```python
from build123d import *

# Parameters (mm, degrees)
F0_W     = 650
F0_H     = 950
F1_DEPTH = 50
F4_DEPTH = 50


with BuildPart() as f1:
    # F0 (on Top) → F1 (new body)
    with BuildSketch(Plane.XY):
        Rectangle(F0_W, F0_H)
    extrude(amount=F1_DEPTH)

    # F3 (on offset) → F4 (join)
    with BuildSketch(Plane.XZ.offset(375)):
        Polygon((0, -158.604646672), (-86.0232526704, -97.1594661932), (-300, -250), (-127.9534946591, -250), align=None)
        Polygon((0, -35.7142857143), (-86.0232526704, -97.1594661932), (0, -158.604646672), (86.0232526704, -97.1594661932), align=None)
        Polygon((50, 0), (0, -35.7142857143), (86.0232526704, -97.1594661932), (222.0465053409, 0), align=None)
        Polygon((-50, 0), (-222.0465053409, 0), (-86.0232526704, -97.1594661932), (0, -35.7142857143), align=None)
        Polygon((86.0232526704, -97.1594661932), (0, -158.604646672), (127.9534946591, -250), (300, -250), align=None)
    extrude(amount=F4_DEPTH)

    # F5: F1 across plane


with BuildPart() as f1_1:
    add(f1.part)
    add(f1.part.mirror(Plane.XZ))


solid = f1_1.part
```
Geometry check sheet. Reference: the model listing, model coordinates, mm. A direction names the side the tool comes from. Give positions to 0.01 mm unless a question says otherwise; leave off trailing zeros. Loops run counter-clockwise (first coordinate to the right, second up) from the corner with the lowest first, then second, coordinate; pieces in that order, holes last. Notation, with made-up numbers: M -7.5,22 L 21.5,22 A36 ccw 21.5,60 Z; hole C -25.5,81.5 d7. An arc over 180 degrees is marked long. Write item = value, one per line. Start each with the question number.
1. Section check B-B, the plane x = -244. Enter the section's corners in (y, z).
2. Go/stop test with flat-tipped pins: P1, Ø2, axis at x = -113, z = -186.5, coming from the -Y side; P2, Ø6, axis at x = 168, y = 4.5, coming from the -Z side; P3, Ø1, axis at x = -116.5, z = -10.5, coming from the +Y side. Record where each tip stops, or that it passes through.
3. Section check C-C, the plane z = -210. Enter the section's corners in (x, y).
4. Tool access check on faces 1 (the face through (-4, 425, -123)), 2 (the face through (63.08, 399.65, -203.66)), 3 (the face through (-191.5, 399.6, -172.5)). Record the directions out of +Z, -Z, +X, -X, +Y, -Y that give a thin tool (end or side, any length) a straight path to the whole face; none if there is none.
5. Thickness scan on probe 1 along Y at (x, z) = (77, -100.5); probe 2 along Z at (x, y) = (-136, -69); probe 3 along Z at (x, y) = (-108.5, -396). Record the ranges inside material, lowest first.
6. Draft check along Z on faces 4 (the face through (-64.87, -399.65, -204.94)), 5 (the face through (-4, -425, -123)), 6 (the face through (153.08, 399.65, -49.26)). Enter one of: +Z half, -Z half, draft (parallel to the pull), parting line (faces both ways), or undercut.
7. Section check A-A, the plane z = -65.5. Enter the section's corners in (x, y).
8. Section check D-D, the plane y = -270. Enter the section's corners in (x, z), plus the area to 3 significant figures.
Values follow:
q1.outline = M -475,0 L 475,0 L 475,50 L -475,50 Z; M -425,-250 L -375,-250 L -375,-210 L -425,-210 Z; M 375,-250 L 425,-250 L 425,-210 L 375,-210 Z
q2.P1 = -425
q2.P2 = 0
q2.P3 = 425
q3.outline = M -244,-425 L -71.95,-425 L -71.95,-375 L -244,-375 Z; M -244,375 L -71.95,375 L -71.95,425 L -244,425 Z; M 71.95,-425 L 244,-425 L 244,-375 L 71.95,-375 Z; M 71.95,375 L 244,375 L 244,425 L 71.95,425 Z
q4.face_1 = -Z, +X, -X, +Y
q4.face_2 = -Z, +Y, -Y
q4.face_3 = -X, +Y, -Y
q5.probe_1 = -425 to -375, 375 to 425
q5.probe_2 = 0 to 50
q5.probe_3 = -236.1 to -113.21, -81.1 to 50
q6.face_4 = -Z half
q6.face_5 = draft
q6.face_6 = undercut
q7.outline = M -130.35,-425 L 130.35,-425 L 130.35,-375 L -130.35,-375 Z; M -130.35,375 L 130.35,375 L 130.35,425 L -130.35,425 Z
q8.outline = M -325,0 L 325,0 L 325,50 L -325,50 Z
q8.area = 32,500 mm^2
